Work out the finished part from the listing and answer in its coordinate system (mm). Face numbers are marked on the shaded views. A direction names the side the tool comes from. Round coordinates to 2 decimals unless told otherwise and drop trailing zeros. Loops run counter-clockwise (first coordinate to the right, second up) from the corner with the lowest first, then second, coordinate; pieces in that order, holes last.
```python
from build123d import *

# Parameters (mm, degrees)
SKETCH1_W               = 130.175
SKETCH1_H               = 110.236
SKETCH1_R               = 1.5875
SKETCH1_R_2             = 5.08
BOSS_EXTRUDE1_DEPTH     = 12.7
CUT_EXTRUDE1_DEPTH      = 87.230311261
CUT_EXTRUDE1_DEPTH_BACK = 87.230311261
SKETCH2_OUTSIDE_W       = 166.385
SKETCH2_OUTSIDE_H       = 146.446


with BuildPart() as part:
    # Sketch1 → Boss-Extrude1 (new body)
    with BuildSketch(Plane(origin=(0, 0, 0), x_dir=(1, 0, 0), z_dir=(0, 1, 0))):
        Rectangle(SKETCH1_W, SKETCH1_H)
        with Locations(Location((-52.3875, 21.59, 0), (0, 0, 270))):
            Circle(SKETCH1_R, mode=Mode.SUBTRACT)
        with Locations(Location((52.3875, 21.59, 0), (0, 0, 270))):
            Circle(SKETCH1_R, mode=Mode.SUBTRACT)
        with Locations(Location((52.3875, -21.59, 0), (0, 0, 270))):
            Circle(SKETCH1_R, mode=Mode.SUBTRACT)
        with Locations(Location((-52.3875, -21.59, 0), (0, 0, 270))):
            Circle(SKETCH1_R, mode=Mode.SUBTRACT)
        with Locations(Location((-42.418, 42.418, 0), (0, 0, 270))):
            Circle(SKETCH1_R_2, mode=Mode.SUBTRACT)
        with Locations(Location((42.418, 42.418, 0), (0, 0, 270))):
            Circle(SKETCH1_R_2, mode=Mode.SUBTRACT)
        with Locations(Location((42.418, -42.418, 0), (0, 0, 270))):
            Circle(SKETCH1_R_2, mode=Mode.SUBTRACT)
        with Locations(Location((-42.418, -42.418, 0), (0, 0, 270))):
            Circle(SKETCH1_R_2, mode=Mode.SUBTRACT)
    extrude(amount=BOSS_EXTRUDE1_DEPTH)

    # Sketch2 outside → Cut-Extrude1 (cut, two sides: drawn at the far end of the back side and taken through both)
    # profile 1 of 9: a face of its own
    with BuildSketch(Plane(origin=(0, 12.7, 0), x_dir=(1, 0, 0), z_dir=(0, 1, 0)).offset(-CUT_EXTRUDE1_DEPTH_BACK)):
        with Locations((-0.0005, 0)):
            Rectangle(SKETCH2_OUTSIDE_W, SKETCH2_OUTSIDE_H)
        with BuildLine():
            Line((42.418, 50.038), (-42.418, 50.038))
            ThreePointArc((-42.418, 50.038), (-46.479726634, 48.865230161), (-49.291198546, 45.707915158))
            Line((-49.291198546, 45.707915158), (-59.260698546, 24.879915158))
            ThreePointArc((-59.260698546, 24.879915158), (-59.818454613, 23.276805721), (-60.0075, 21.59))
            Line((-60.0075, 21.59), (-60.0075, -21.59))
            ThreePointArc((-60.0075, -21.59), (-59.818454613, -23.276805721), (-59.260698546, -24.879915158))
            Line((-59.260698546, -24.879915158), (-49.291198546, -45.707915158))
            ThreePointArc((-49.291198546, -45.707915158), (-46.479726634, -48.865230161), (-42.418, -50.038))
            Line((-42.418, -50.038), (42.418, -50.038))
            ThreePointArc((42.418, -50.038), (46.479726634, -48.865230161), (49.291198546, -45.707915158))
            Line((49.291198546, -45.707915158), (59.260698546, -24.879915158))
            ThreePointArc((59.260698546, -24.879915158), (59.818454613, -23.276805721), (60.0075, -21.59))
            Line((60.0075, -21.59), (60.0075, 21.59))
            ThreePointArc((60.0075, 21.59), (59.818454613, 23.276805721), (59.260698546, 24.879915158))
            Line((59.260698546, 24.879915158), (49.291198546, 45.707915158))
            ThreePointArc((49.291198546, 45.707915158), (46.479726634, 48.865230161), (42.418, 50.038))
        make_face(mode=Mode.SUBTRACT)
    # profile 2 of 9: a face of its own
    with BuildSketch(Plane(origin=(0, 12.7, 0), x_dir=(1, 0, 0), z_dir=(0, 1, 0)).offset(-CUT_EXTRUDE1_DEPTH_BACK)):
        with BuildLine():
            Line((-27.087743879, -37.338), (27.087743879, -37.338))
            ThreePointArc((27.087743879, -37.338), (28.261070885, -36.554007959), (27.985769491, -35.169974388))
            Line((27.985769491, -35.169974388), (0.898025612, -8.082230509))
            ThreePointArc((0.898025612, -8.082230509), (0, -7.710256121), (-0.898025612, -8.082230509))
            Line((-0.898025612, -8.082230509), (-27.985769491, -35.169974388))
            ThreePointArc((-27.985769491, -35.169974388), (-28.261070885, -36.554007959), (-27.087743879, -37.338))
        make_face()
    # profile 3 of 9: a face of its own
    with BuildSketch(Plane(origin=(0, 12.7, 0), x_dir=(1, 0, 0), z_dir=(0, 1, 0)).offset(-CUT_EXTRUDE1_DEPTH_BACK)):
        with BuildLine():
            Line((-44.245555664, -23.729025589), (-27.442482896, -16.804122872))
            ThreePointArc((-27.442482896, -16.804122872), (-25.901976239, -17.273686348), (-26.060547132, -18.876342235))
            Line((-26.060547132, -18.876342235), (-39.665944234, -32.481739337))
            ThreePointArc((-39.665944234, -32.481739337), (-40.778186169, -32.835516971), (-41.709502937, -32.132032918))
            Line((-41.709502937, -32.132032918), (-44.907178603, -25.451538533))
            ThreePointArc((-44.907178603, -25.451538533), (-44.947197717, -24.447844803), (-44.245555664, -23.729025589))
        make_face()
    # profile 4 of 9: a face of its own
    with BuildSketch(Plane(origin=(0, 12.7, 0), x_dir=(1, 0, 0), z_dir=(0, 1, 0)).offset(-CUT_EXTRUDE1_DEPTH_BACK)):
        with BuildLine():
            Line((-45.553589848, -13.279107107), (-16.181373616, -1.174193751))
            ThreePointArc((-16.181373616, -1.174193751), (-15.395283768, 0), (-16.181373616, 1.174193751))
            Line((-16.181373616, 1.174193751), (-45.553589848, 13.279107107))
            ThreePointArc((-45.553589848, 13.279107107), (-46.744017554, 13.160248823), (-47.3075, 12.104913356))
            Line((-47.3075, 12.104913356), (-47.3075, -12.104913356))
            ThreePointArc((-47.3075, -12.104913356), (-46.744017554, -13.160248823), (-45.553589848, -13.279107107))
        make_face()
    # profile 5 of 9: a face of its own
    with BuildSketch(Plane(origin=(0, 12.7, 0), x_dir=(1, 0, 0), z_dir=(0, 1, 0)).offset(-CUT_EXTRUDE1_DEPTH_BACK)):
        with BuildLine():
            Line((-44.245555664, 23.729025589), (-27.442482896, 16.804122872))
            ThreePointArc((-27.442482896, 16.804122872), (-25.901976239, 17.273686348), (-26.060547132, 18.876342235))
            Line((-26.060547132, 18.876342235), (-39.665944234, 32.481739337))
            ThreePointArc((-39.665944234, 32.481739337), (-40.778186169, 32.835516971), (-41.709502937, 32.132032918))
            Line((-41.709502937, 32.132032918), (-44.907178603, 25.451538533))
            ThreePointArc((-44.907178603, 25.451538533), (-44.947197717, 24.447844803), (-44.245555664, 23.729025589))
        make_face()
    # profile 6 of 9: a face of its own
    with BuildSketch(Plane(origin=(0, 12.7, 0), x_dir=(1, 0, 0), z_dir=(0, 1, 0)).offset(-CUT_EXTRUDE1_DEPTH_BACK)):
        with BuildLine():
            Line((0.898025612, 8.082230509), (27.985769491, 35.169974388))
            ThreePointArc((27.985769491, 35.169974388), (28.261070885, 36.554007959), (27.087743879, 37.338))
            Line((27.087743879, 37.338), (-27.087743879, 37.338))
            ThreePointArc((-27.087743879, 37.338), (-28.261070885, 36.554007959), (-27.985769491, 35.169974388))
            Line((-27.985769491, 35.169974388), (-0.898025612, 8.082230509))
            ThreePointArc((-0.898025612, 8.082230509), (0, 7.710256121), (0.898025612, 8.082230509))
        make_face()
    # profile 7 of 9: a face of its own
    with BuildSketch(Plane(origin=(0, 12.7, 0), x_dir=(1, 0, 0), z_dir=(0, 1, 0)).offset(-CUT_EXTRUDE1_DEPTH_BACK)):
        with BuildLine():
            Line((27.442482896, 16.804122872), (44.245555664, 23.729025589))
            ThreePointArc((44.245555664, 23.729025589), (44.947197717, 24.447844803), (44.907178603, 25.451538533))
            Line((44.907178603, 25.451538533), (41.709502937, 32.132032918))
            ThreePointArc((41.709502937, 32.132032918), (40.778186169, 32.835516971), (39.665944234, 32.481739337))
            Line((39.665944234, 32.481739337), (26.060547132, 18.876342235))
            ThreePointArc((26.060547132, 18.876342235), (25.901976239, 17.273686348), (27.442482896, 16.804122872))
        make_face()
    # profile 8 of 9: a face of its own
    with BuildSketch(Plane(origin=(0, 12.7, 0), x_dir=(1, 0, 0), z_dir=(0, 1, 0)).offset(-CUT_EXTRUDE1_DEPTH_BACK)):
        with BuildLine():
            Line((16.181373616, 1.174193751), (45.553589848, 13.279107107))
            ThreePointArc((45.553589848, 13.279107107), (46.744017554, 13.160248823), (47.3075, 12.104913356))
            Line((47.3075, 12.104913356), (47.3075, -12.104913356))
            ThreePointArc((47.3075, -12.104913356), (46.744017554, -13.160248823), (45.553589848, -13.279107107))
            Line((45.553589848, -13.279107107), (16.181373616, -1.174193751))
            ThreePointArc((16.181373616, -1.174193751), (15.395283768, 0), (16.181373616, 1.174193751))
        make_face()
    # profile 9 of 9: a face of its own
    with BuildSketch(Plane(origin=(0, 12.7, 0), x_dir=(1, 0, 0), z_dir=(0, 1, 0)).offset(-CUT_EXTRUDE1_DEPTH_BACK)):
        with BuildLine():
            Line((26.060547132, -18.876342235), (39.665944234, -32.481739337))
            ThreePointArc((39.665944234, -32.481739337), (40.778186169, -32.835516971), (41.709502937, -32.132032918))
            Line((41.709502937, -32.132032918), (44.907178603, -25.451538533))
            ThreePointArc((44.907178603, -25.451538533), (44.947197717, -24.447844803), (44.245555664, -23.729025589))
            Line((44.245555664, -23.729025589), (27.442482896, -16.804122872))
            ThreePointArc((27.442482896, -16.804122872), (25.901976239, -17.273686348), (26.060547132, -18.876342235))
        make_face()
    extrude(amount=CUT_EXTRUDE1_DEPTH + CUT_EXTRUDE1_DEPTH_BACK, mode=Mode.SUBTRACT)


solid = part.part
```
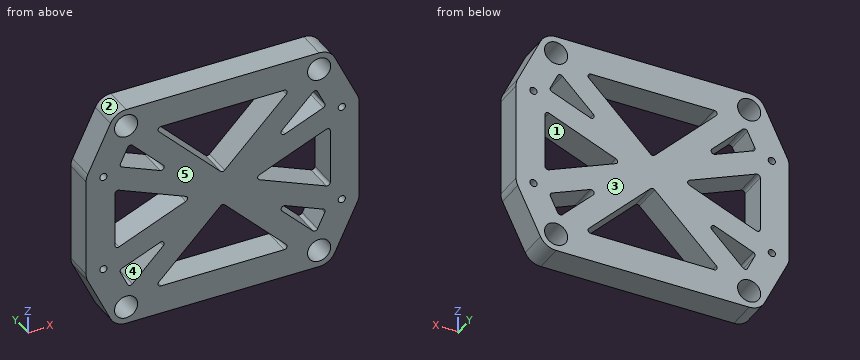
1. Consider probe 1 along Z at (x, y) = (-37, 0.5); probe 2 along X at (y, z) = (7.25, 41.5); probe 3 along Z at (x, y) = (30, 1.75). Determine where each line is inside the solid, lowest interval first.
Answer key:
probe 1: z = -50.04 to -29.82, -20.74 to -9.75, 9.75 to 20.74, 29.82 to 50.04
probe 2: x = -51.31 to -47.41, -37.42 to 37.42, 47.41 to 51.31
probe 3: z = -50.04 to -22.82, -17.86 to -6.87, 6.87 to 17.86, 22.82 to 50.04
2. Find section D-D (y = 2.5). Give the number of separate pieces and of enclosed holes in the cut face, then the cut area to 3 significant figures.
Answer key:
separate pieces: 1
enclosed holes: 16
area: 7,680 mm2
3. Find section C-C (z = 27.5). Write down the section's boundary in (x, y).
Answer key:
outline: (-58.01, 0) - (-43.93, 0) - (-43.93, 12.7) - (-58.01, 12.7) - close; (-34.68, 0) - (-20.32, 0) - (-20.32, 12.7) - (-34.68, 12.7) - close; (20.32, 0) - (34.68, 0) - (34.68, 12.7) - (20.32, 12.7) - close; (43.93, 0) - (58.01, 0) - (58.01, 12.7) - (43.93, 12.7) - close
4. Given pin 1 (8 mm diameter, centred on x = 42.418, z = 42.418, fed in from -Y), flat-ended and moving along its own axis, determine where the tip first touches the part or whether it passes through.
Answer key:
pin 1: passes through
5. Determine the mould class of the marked faces 1, 2 and 3 for opening direction X: +X half, -X half, draft (parallel to the pull), parting line (faces both ways), or undercut.
Answer key:
face 1: undercut
face 2: -X half
face 3: draft
6. Find section B-B (x = -23). Write down the section's boundary in (y, z), then the cut area to 3 significant figures.
Answer key:
outline: (0, -50.04) - (12.7, -50.04) - (12.7, -37.34) - (0, -37.34) - close; (0, -30.18) - (12.7, -30.18) - (12.7, -3.98) - (0, -3.98) - close; (0, 3.98) - (12.7, 3.98) - (12.7, 30.18) - (0, 30.18) - close; (0, 37.34) - (12.7, 37.34) - (12.7, 50.04) - (0, 50.04) - close
area: 988 mm2
7. Which of the six approach directions +Z, -Z, +X, -X, +Y, -Y give full straight-line access (tool end or side, diameter ignored) to the marked faces 4 and 5?
Answer key:
face 4: +Y, -Y
face 5: +Z, -Z, +X, -X, -Y
8. Find section A-A (x = 9.5). Write down the section's boundary in (y, z), then the cut area to 3 significant figures.
Answer key:
outline: (0, -50.04) - (12.7, -50.04) - (12.7, -37.34) - (0, -37.34) - close; (0, -16.68) - (12.7, -16.68) - (12.7, 16.68) - (0, 16.68) - close; (0, 37.34) - (12.7, 37.34) - (12.7, 50.04) - (0, 50.04) - close
area: 746 mm2
